The listing builds one solid part. Answer for the finished solid, in the listing's coordinates (mm). A direction names the side the tool comes from. Coordinates: 2 decimals unless noted, no trailing zeros. Write each loop counter-clockwise with the first axis right and the second up, starting at its lowest first coordinate (ties: lowest second). Pieces come first, ordered by that corner, then holes. Notation, with made-up numbers: M 53.5,57 L 86.5,57 A38 ccw 86.5,95 Z; hole C 37,10.25 d3. An arc over 180 degrees is marked long. Answer as CSV lines item,"result".
```python
from build123d import *

# Parameters (mm, degrees)
SKETCH1_R           = 20
SKETCH1_R_2         = 9
BOSS_EXTRUDE1_DEPTH = 21
SKETCH1_3_W         = 16
SKETCH1_3_H         = 120
BOSS_EXTRUDE2_DEPTH = 16
BOSS_EXTRUDE3_DEPTH = 16
BOSS_EXTRUDE4_START = 9
SKETCH2_3_R         = 30
SKETCH2_3_R_2       = 15
BOSS_EXTRUDE4_DEPTH = 25
GURT_R              = 20
GURT_R_2            = 8
BOSS_EXTRUDE5_DEPTH = 12
BOSS_EXTRUDE6_DEPTH = 6
BOSS_EXTRUDE7_DEPTH = 5


with BuildPart() as part:
    # Sketch1 → Boss-Extrude1 (new body)
    with BuildSketch(Plane(origin=(0, 0, 0), x_dir=(1, 0, 0), z_dir=(0, 1, 0))):
        with Locations(Location((0, 0, 0), (0, 0, 90))):
            Circle(SKETCH1_R)
        with Locations(Location((0, 0, 0), (0, 0, 90))):
            Circle(SKETCH1_R_2, mode=Mode.SUBTRACT)
    extrude(amount=BOSS_EXTRUDE1_DEPTH)

    # Sketch1_3 → Boss-Extrude2 (add)
    with BuildSketch(Plane(origin=(0, 0, 0), x_dir=(1, 0, 0), z_dir=(0, 1, 0))):
        with BuildLine():
            Line((120, 0), (20, 0))
            ThreePointArc((20, 0), (11.756842217, -16.179513623), (-6.177666108, -19.021998882))
            Line((-6.177666108, -19.021998882), (120, -60))
            Line((120, -60), (120, 0))
        make_face()
        with BuildLine():
            ThreePointArc((-6.177666108, 19.021998882), (11.756842217, 16.179513623), (20, 0))
            Line((20, 0), (120, 0))
            Line((120, 0), (120, 60))
            Line((120, 60), (-6.177666108, 19.021998882))
        make_face()
        with Locations((128, 0)):
            Rectangle(SKETCH1_3_W, SKETCH1_3_H)
    extrude(amount=BOSS_EXTRUDE2_DEPTH)

    # Sketch2 → Boss-Extrude3 (add)
    with BuildSketch(Plane(origin=(136, 0, 0), x_dir=(0, 0, -1), z_dir=(1, 0, 0))):
        with BuildLine():
            Line((-28.597626566, 115.065084378), (-60, 16))
            Line((-60, 16), (60, 16))
            Line((60, 16), (28.597626566, 115.065084378))
            ThreePointArc((28.597626566, 115.065084378), (29.64733375, 110.586458493), (30, 106))
            ThreePointArc((30, 106), (-4.586458493, 76.35266625), (-28.597626566, 115.065084378))
        make_face()
    extrude(amount=-BOSS_EXTRUDE3_DEPTH)

    # Sketch2_3 → Boss-Extrude4 (add)
    with BuildSketch(Plane(origin=(136, 0, 0), x_dir=(0, 0, -1), z_dir=(1, 0, 0)).offset(BOSS_EXTRUDE4_START)):
        with Locations(Location((0, 106, 0), (0, 0, 162.412046226))):
            Circle(SKETCH2_3_R)
        with Locations((0, 106)):
            Circle(SKETCH2_3_R_2, mode=Mode.SUBTRACT)
    extrude(amount=-BOSS_EXTRUDE4_DEPTH)



with BuildPart() as body_2:
    # gurt → Boss-Extrude5 (new, symmetric)
    with BuildSketch(Plane.XY):
        with Locations((70, 61)):
            Circle(GURT_R)
        with Locations((70, 61)):
            Circle(GURT_R_2, mode=Mode.SUBTRACT)
    extrude(amount=BOSS_EXTRUDE5_DEPTH, both=True)


with BuildPart() as part_1:
    add(part.part)

    add(body_2.part)  # Boss-Extrude6 merges body 2
    # gurt_4 → Boss-Extrude6 (add, symmetric)
    with BuildSketch(Plane.XY):
        with BuildLine():
            Line((120, 81), (70, 81))
            ThreePointArc((70, 81), (84.142135624, 75.142135624), (90, 61))
            ThreePointArc((90, 61), (64.275108868, 41.83686817), (53.277437847, 71.970684347))
            Line((53.277437847, 71.970684347), (19.838585367, 21))
            Line((19.838585367, 21), (19.838585367, 16))
            Line((19.838585367, 16), (120, 16))
            Line((120, 16), (120, 81))
        make_face()
    extrude(amount=BOSS_EXTRUDE6_DEPTH, both=True)

    # Sketch4 → Boss-Extrude7 (add)
    with BuildSketch(Plane(origin=(0, 16, 0), x_dir=(1, 0, 0), z_dir=(0, 1, 0))):
        Polygon((19.838585367, 2.535849097), (19.838585367, 6), (18.936316569, 6), align=None)
        Polygon((19.838585367, -6), (18.936316569, -6), (19.838585367, -2.535849097), align=None)
    extrude(amount=BOSS_EXTRUDE7_DEPTH)


solid = part_1.part
```
Q1. Flat-ended cylindrical pins translate along their axes: pin 1 Ø18.5 at (x, y) = (70, 61) entering from -Z; pin 2 Ø19.5 at (x, y) = (76, 58.5) entering from +Z; pin 3 Ø3.5 at (x, z) = (87, -2) entering from +Y. Find the tip coordinate at first contact, or state that the pin passes through.
Output:
pin 1,"z = -12"
pin 2,"z = 12"
pin 3,"y = 81"
Q2. Find section A-A (z = 0). Give the vertices of the cut face in (x, y), and give its area (3 significant figures).
Output:
outline,"M -20,0 L -9,0 L -9,21 L -20,21 Z; M 9,0 L 136,0 L 136,76 L 145,76 L 145,91 L 120,91 L 120,81 L 70,81 A20 ccw 53.28,71.97 L 19.84,21 L 9,21 Z; M 120,121 L 145,121 L 145,136 L 120,136 Z; hole C 70,61 d16"
area,"9,140 mm2"
Q3. Find section C-C (y = 61). Give the vertices of the cut face in (x, z), and give its area (3 significant figures).
Output:
outline,"M 46.08,-6 L 50,-6 L 50,-12 L 62,-12 L 62,12 L 50,12 L 50,6 L 46.08,6 Z; M 78,-12 L 90,-12 L 90,-6 L 120,-6 L 120,-45.74 L 136,-45.74 L 136,45.74 L 120,45.74 L 120,6 L 90,6 L 90,12 L 78,12 Z"
area,"2,450 mm2"
Q4. For faces 1 (the cylindrical face through (135.453, 135.554, 5.154)), 2 (the flat face through (70, 52, -12)), 3 (the flat face through (81, 41, -6)), determine the directions among +Z, -Z, +X, -X, +Y, -Y from which every point of the face is accessible in a straight line to the end or side of a thin tool.
Output:
face 1,"+X"
face 2,"-Z, -X, +Y"
face 3,"-Z"
Q5. The mould has two halves that part along X. Classify faces 4 (the flat face through (136, 33, 1)), 5 (the cylindrical face through (-2.703, 10.353, -8.584)), 6 (the flat face through (128, 8, -60)), 7 (the flat face through (57.8, 7.9, -39.8)): pulls with the +X half, pulls with the -X half, needs draft (parallel to the pull), parting line crosses it, or undercut.
Output:
face 4,"pulls with the +X half"
face 5,"undercut"
face 6,"needs draft"
face 7,"pulls with the -X half"
Q6. Straight lines are drawn through the part: line 1 (Y direction, x = 70, z = 6.5); line 2 (X direction, y = 5, z = 0); line 3 (Z direction, x = 114, y = 61). For each, find the intervals that lie inside material, in ascending order.
Output:
line 1,"0 to 16, 41 to 53, 69 to 81"
line 2,"-20 to -9, 9 to 136"
line 3,"-6 to 6"
Q7. Find section B-B (x = 122.5). Give the vertices of the cut face in (y, z).
Output:
outline,"M 0,-60 L 16,-60 L 115.07,-28.6 A30 ccw 115.07,28.6 L 16,60 L 0,60 Z; hole C 106,0 d30"
Q8. Find section D-D (x = 0). Give the vertices of the cut face in (y, z).
Output:
outline,"M 0,-21.03 L 16,-21.03 L 16,-20 L 21,-20 L 21,-9 L 0,-9 Z; M 0,9 L 21,9 L 21,20 L 16,20 L 16,21.03 L 0,21.03 Z"
